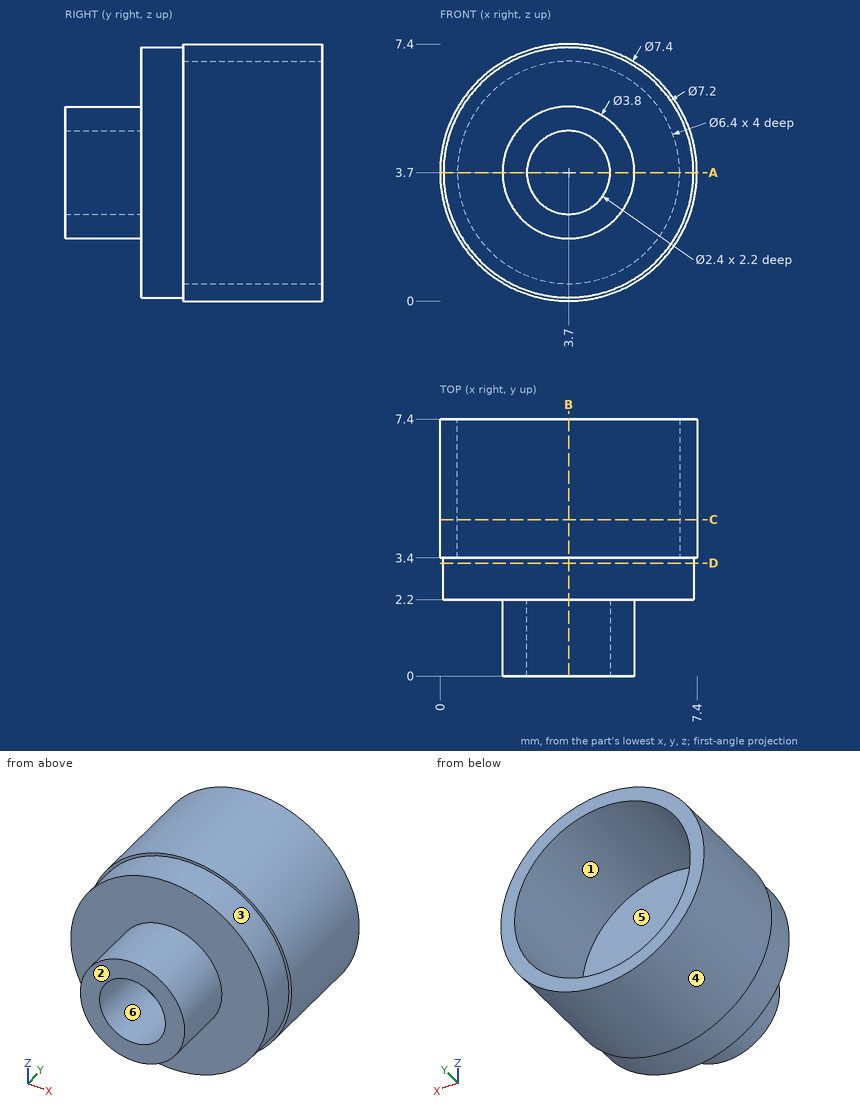
Print and shaded views of the part. All mm, measured from the part's lowest x, y and z. A direction names the side the tool comes from. Coordinates: 2 decimals unless noted, no trailing zeros. Order: outer loops, then holes, each group sorted by start corner. A loop starts at its lowest first (then second) coordinate and runs counter-clockwise, first axis right, second up. Notation, with made-up numbers: (-17, 10) -> (-2, 10) arc R7 cw to (-2, 18) -> close; hole circle Ø9 at (46, 65). An arc over 180 degrees is marked (long way). Use one line per item in the form item = value. Start each with the question number.
1) Tool access for the marked faces 4, 5 and 6: list every direction of +Z, -Z, +X, -X, +Y, -Y with a clear straight run to the whole face (end or side of a thin tool).
2) Band-saw the part on B-B on x = 3.7. Give the cut face in (y, z), then the cut area to 3 significant figures.
3) Drop flat-ended pins along their axis: pin 1 (1 mm diameter, centred on x = 4, z = 4, fed in from +Y); pin 2 (1.5 mm diameter, centred on x = 1, y = 3, fed in from -Z); pin 3 (1.4 mm diameter, centred on x = 3.7, z = 3.7, fed in from -Y). Give the stop position or say it passes through.
4) Band-saw the part on D-D on y = 3.25. Give the cut face in (x, z), then the cut area to 3 significant figures.
5) Pull direction X, two halves, no side cores. Call the marked faces 1, 2 and 3: +X half, -X half, draft (parallel to the pull), parting line (faces both ways), or undercut.
6) Band-saw the part on C-C on y = 4.5. Give the cut face in (x, z), then the cut area to 3 significant figures.
7) Drill centre lines: L1, parallel to Z at x = 3.7, y = 5.3; L2, parallel to Z at x = 3.7, y = 1.55; L3, parallel to Y at x = 1.25, z = 3.5. Where is each one in solid material? Low to high. Write a range as [from, to].
8) Band-saw the part on A-A on z = 3.7. Give the cut face in (x, y).
Entries:
q1.face_4 = +Y, -Y
q1.face_5 = +Y
q1.face_6 = -Y
q2.outline = (0, 1.8) -> (2.2, 1.8) -> (2.2, 0.1) -> (3.4, 0.1) -> (3.4, 0) -> (7.4, 0) -> (7.4, 0.5) -> (3.4, 0.5) -> (3.4, 6.9) -> (7.4, 6.9) -> (7.4, 7.4) -> (3.4, 7.4) -> (3.4, 7.3) -> (2.2, 7.3) -> (2.2, 5.6) -> (0, 5.6) -> (0, 4.9) -> (2.2, 4.9) -> (2.2, 2.5) -> (0, 2.5) -> close
q2.area = 15.7 mm2
q3.pin_1 = 3.4
q3.pin_2 = 0.63
q3.pin_3 = 2.2
q4.outline = circle Ø7.2 at (3.7, 3.7)
q4.area = 40.7 mm2
q5.face_1 = undercut
q5.face_2 = draft
q5.face_3 = parting line
q6.outline = circle Ø7.4 at (3.7, 3.7); hole circle Ø6.4 at (3.7, 3.7)
q6.area = 10.8 mm2
q7.L1 = [0, 0.5], [6.9, 7.4]
q7.L2 = [1.8, 2.5], [4.9, 5.6]
q7.L3 = [2.2, 3.4]
q8.outline = (0, 3.4) -> (0.1, 3.4) -> (0.1, 2.2) -> (1.8, 2.2) -> (1.8, 0) -> (2.5, 0) -> (2.5, 2.2) -> (4.9, 2.2) -> (4.9, 0) -> (5.6, 0) -> (5.6, 2.2) -> (7.3, 2.2) -> (7.3, 3.4) -> (7.4, 3.4) -> (7.4, 7.4) -> (6.9, 7.4) -> (6.9, 3.4) -> (0.5, 3.4) -> (0.5, 7.4) -> (0, 7.4) -> close
